Source: CAD feature listing. Evaluate the final solid. Frame: model axes, mm. A direction names the side the tool comes from. Round coordinates to 2 decimals unless told otherwise and drop trailing zeros. Order: outer loops, then holes, each group sorted by start corner. A loop starts at its lowest first (then second) coordinate and runs counter-clockwise, first axis right, second up. Notation, with made-up numbers: (30, 5) -> (73, 5) arc R17 cw to (73, 28) -> close; hole circle Ø11 at (83, 32.25). An arc over 180 degrees is marked (long way). One line per item, written item: value. Start each with the question number.
1) Section B-B (x = 0). Return the cut outline in (y, z).
2) Mould query, pull axis X, two halves, no side actions, for faces 1 (the face through (1, -33, -44.5)), 2 (the face through (90.49, -30.93, -44.65)), 3 (the face through (0, -61, 46)). Classes: pulls with the +X half, pulls with the -X half, needs draft (parallel to the pull), parting line crosses it, or undercut.
3) Section C-C (y = -37). Return the cut outline in (x, z).
4) Section D-D (z = 14.5). Return the cut outline in (x, y).
5) Ray query, L1, parallel to Z at x = 84, y = -32; L2, parallel to Z at x = 29, y = -36.5; L3, parallel to X at y = -52, z = 6.5. Return the intervals inside material, ascending.
6) Section A-A (y = -25). Return the cut outline in (x, z), and give its area (3 significant figures).
7) Pin query (flat end, axial travel): P1, Ø10, axis at x = -84.5, z = 38.5, coming from the +Y side; P2, Ø4, axis at x = 41.5, z = 7.5, coming from the -Y side. Return the tip coordinate at first contact, or that it passes through.
8) Reachability of faces 4 (the face through (-87, -10, -41)), 5 (the face through (-1, -30, -47.5)), 6 (the face through (90.5, -33, 0)) from +Z, -Z, +X, -X, +Y, -Y: full face, straight path, thin tool, end or side. Return the list, or none.
```python
from build123d import *

# Parameters (mm, degrees)
F0_W     = 187
F0_H     = 95
F0_R     = 3
F1_DEPTH = 6
F2_W     = 187
F2_H     = 95
F2_R     = 3
F3_DEPTH = 55
F4_R     = 10
F5_R     = 5.5
F6_DEPTH = 10
F7_R     = 3
F8_DEPTH = 25


with BuildPart() as f1:
    # F0 (on Front) → F1 (new body)
    with BuildSketch(Plane.XZ):
        Rectangle(F0_W, F0_H)
        with Locations((-84.5, -38.5)):
            Circle(F0_R, mode=Mode.SUBTRACT)
        with Locations((84.5, -38.5)):
            Circle(F0_R, mode=Mode.SUBTRACT)
        with Locations((-84.5, 38.5)):
            Circle(F0_R, mode=Mode.SUBTRACT)
        with Locations((84.5, 38.5)):
            Circle(F0_R, mode=Mode.SUBTRACT)
    extrude(amount=F1_DEPTH)

    # F2 (on face) → F3 (join)
    with BuildSketch(Plane.XZ.offset(6)):
        Rectangle(F2_W, F2_H)
        with Locations((-84.5, -38.5)):
            Circle(F2_R, mode=Mode.SUBTRACT)
        with Locations((84.5, -38.5)):
            Circle(F2_R, mode=Mode.SUBTRACT)
        with BuildLine():
            ThreePointArc((78.479203, 44.5), (78.686333, 32.686563), (90.5, 32.492996))
            Line((90.5, 32.492996), (90.5, -32.487318))
            ThreePointArc((90.5, -32.487318), (78.324787, -32.32468), (78.479203, -44.5))
            Line((78.479203, -44.5), (-78.483447, -44.5))
            ThreePointArc((-78.483447, -44.5), (-78.593686, -32.593646), (-90.5, -32.479203))
            Line((-90.5, -32.479203), (-90.5, 32.479203))
            ThreePointArc((-90.5, 32.479203), (-78.867749, 32.866318), (-78.526316, 44.5))
            Line((-78.526316, 44.5), (78.479203, 44.5))
        make_face(mode=Mode.SUBTRACT)
        with Locations((-84.5, 38.5)):
            Circle(F2_R, mode=Mode.SUBTRACT)
        with Locations((84.5, 38.5)):
            Circle(F2_R, mode=Mode.SUBTRACT)
    extrude(amount=F3_DEPTH)

    # F4
    f4_edges = [f1.edges().sort_by_distance(p)[0] for p in [
        (-93.5, -30.5, -47.5),
        (-93.5, -30.5, 47.5),
        (93.5, -30.5, 47.5),
        (93.5, -30.5, -47.5),
    ]]
    fillet(f4_edges, radius=F4_R)

    # F5 (on face) → F6 (cut)
    with BuildSketch(Plane(origin=(0, 0, 0), x_dir=(-1, 0, 0), z_dir=(0, 1, 0))):
        with Locations((-84.5, 38.5)):
            Circle(F5_R)
        with Locations((-84.5, -38.5)):
            Circle(F5_R)
        with Locations((84.5, -38.5)):
            Circle(F5_R)
        with Locations((84.5, 38.5)):
            Circle(F5_R)
    extrude(amount=-F6_DEPTH, mode=Mode.SUBTRACT)

    # F7 (on face) → F8 (cut)
    with BuildSketch(Plane.XY.offset(47.5)):
        with Locations((0, -25)):
            Circle(F7_R)
    extrude(amount=-F8_DEPTH, mode=Mode.SUBTRACT)


solid = f1.part
```
Findings:
1. outline: (-61, -47.5) -> (0, -47.5) -> (0, 47.5) -> (-22, 47.5) -> (-22, 44.5) -> (-6, 44.5) -> (-6, -44.5) -> (-61, -44.5) -> close; (-61, 44.5) -> (-28, 44.5) -> (-28, 47.5) -> (-61, 47.5) -> close
2. face 1: undercut
2. face 2: pulls with the +X half
2. face 3: needs draft
3. outline: (-93.5, -37.5) arc R10 ccw to (-83.5, -47.5) -> (83.5, -47.5) arc R10 ccw to (93.5, -37.5) -> (93.5, 37.5) arc R10 ccw to (83.5, 47.5) -> (-83.5, 47.5) arc R10 ccw to (-93.5, 37.5) -> close; hole (-90.5, -32.48) arc R8.5 cw to (-78.48, -44.5) -> (78.48, -44.5) arc R8.5 cw (long way) to (90.5, -32.49) -> (90.5, 32.49) arc R8.5 cw to (78.48, 44.5) -> (-78.53, 44.5) arc R8.5 cw to (-90.5, 32.48) -> close; hole circle Ø6 at (-84.5, -38.5); hole circle Ø6 at (-84.5, 38.5); hole circle Ø6 at (84.5, -38.5); hole circle Ø6 at (84.5, 38.5)
4. outline: (-93.5, -61) -> (-90.5, -61) -> (-90.5, -6) -> (90.5, -6) -> (90.5, -61) -> (93.5, -61) -> (93.5, 0) -> (-93.5, 0) -> close
5. L1: -47.49 to -41.46, -35.54 to -29.84, 30.23 to 35.54, 41.46 to 47.49
5. L2: -47.5 to -44.5, 44.5 to 47.5
5. L3: -93.5 to -90.5, 90.5 to 93.5
6. outline: (-93.5, -37.5) arc R10 ccw to (-83.5, -47.5) -> (83.5, -47.5) arc R10 ccw to (93.5, -37.5) -> (93.5, 37.5) arc R10 ccw to (83.5, 47.5) -> (3, 47.5) -> (3, 44.5) -> (78.48, 44.5) arc R8.5 ccw to (90.5, 32.49) -> (90.5, -32.49) arc R8.5 ccw (long way) to (78.48, -44.5) -> (-78.48, -44.5) arc R8.5 ccw to (-90.5, -32.48) -> (-90.5, 32.48) arc R8.5 ccw to (-78.53, 44.5) -> (-3, 44.5) -> (-3, 47.5) -> (-83.5, 47.5) arc R10 ccw to (-93.5, 37.5) -> close; hole circle Ø6 at (-84.5, -38.5); hole circle Ø6 at (-84.5, 38.5); hole circle Ø6 at (84.5, -38.5); hole circle Ø6 at (84.5, 38.5)
6. area: 2,170 mm2
7. P1: y = -10
7. P2: y = -6
8. face 4: +Y
8. face 5: -Z, +X, -X, +Y, -Y
8. face 6: -Y
